Model file for the job. Use its own axes, mm. Coordinates: 2 decimals unless noted, no trailing zeros. Order: outer loops, then holes, each group sorted by start corner. A loop starts at its lowest first (then second) coordinate and runs counter-clockwise, first axis right, second up.
from build123d import *

# Parameters (mm, degrees)
F0_W     = 94.519034
F0_H     = 86.812686
F0_R     = 5.413518
F0_R_2   = 4.626995
F0_R_3   = 6.390639
F0_R_4   = 9.062056
F0_R_5   = 19.480322
F0_R_6   = 4.110136
F0_R_7   = 4.393433
F0_R_8   = 8.620442
F0_R_9   = 7.192681
F0_R_10  = 4.466697
F1_ANGLE = 45


with BuildPart() as f1:
    # F0 (on Front) → F1 (revolve)
    with BuildSketch(Plane.XZ):
        with Locations((-17.815083, 3.718389)):
            Rectangle(F0_W, F0_H)
        with Locations((-53.812075, -27.955186)):
            Circle(F0_R, mode=Mode.SUBTRACT)
        with Locations((-30.148292, -29.630704)):
            Circle(F0_R_2, mode=Mode.SUBTRACT)
        with Locations((11.945384, -26.993094)):
            Circle(F0_R_3, mode=Mode.SUBTRACT)
        with Locations((-4.236709, -16.035384)):
            Circle(F0_R_4, mode=Mode.SUBTRACT)
        with Locations((-29.292393, 7.944192)):
            Circle(F0_R_5, mode=Mode.SUBTRACT)
        with Locations((-57.312123, 32.896079)):
            Circle(F0_R_6, mode=Mode.SUBTRACT)
        with Locations((-41.277222, 36.766876)):
            Circle(F0_R_7, mode=Mode.SUBTRACT)
        with Locations((5.348549, 12.50712)):
            Circle(F0_R_8, mode=Mode.SUBTRACT)
        with Locations((-7.967654, 32.40367)):
            Circle(F0_R_9, mode=Mode.SUBTRACT)
        with Locations((10.63888, 32.776453)):
            Circle(F0_R_10, mode=Mode.SUBTRACT)
    revolve(axis=Axis((29.444434, 0, 3.718389), (0, 0, -1)), revolution_arc=F1_ANGLE)


solid = f1.part
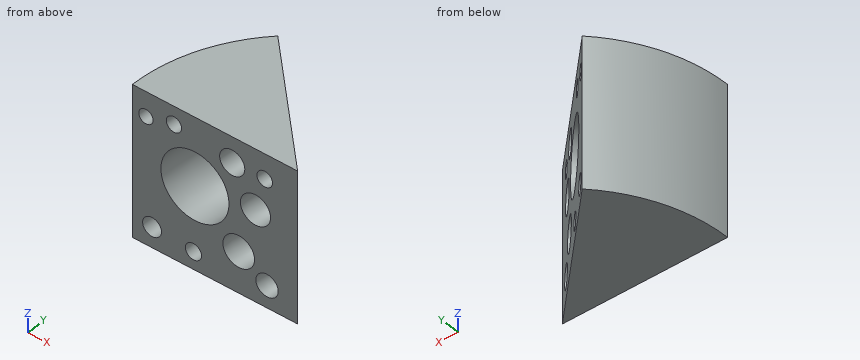
Q1. Probe line 1 (Z direction, x = 10, y = 4.5); line 2 (Z direction, x = 5, y = 9.5); line 3 (Z direction, x = -13, y = 9). List the from-to ranges inside material, lowest first.
Established:
line 1: z = -39.69 to -32.89, -21.09 to 4.94, 20.07 to 28.46, 37.09 to 47.12
line 2: z = -39.69 to -21.19, -10.88 to 4.15, 20.86 to 47.12
line 3: z = -39.69 to -4.05, 19.94 to 28.4, 36.41 to 47.12
Q2. Drop flat-ended pins along their axis: P1, Ø4, axis at y = 50.5, z = 6.5, coming from the +X side; P2, Ø5, axis at y = 19.5, z = 33, coming from the -X side; P3, Ø1.5, axis at x = -41, z = 17, coming from the +Y side. Give the stop position or say it passes through.
Established:
P1: stops at x = -28.45
P2: stops at x = -63.53
P3: stops at y = 63.85
Q3. Cut at D-D, the plane x = -23.5. Count the separate pieces of the cut face and the enclosed holes in it, plus the area to 3 significant figures.
Established:
separate pieces: 2
enclosed holes: 1
area: 2,440 mm2
Q4. Cut at A-A, the plane z = 14.5. List the corners of the cut face in (x, y), plus the area to 3 significant figures.
Established:
outline: (-65.07, 0) - (-47.64, 0) arc R77.08 cw to (-25.06, 54.5) - (-37.39, 66.84) arc R94.52 ccw to start; (-10.95, 0) - (-3.04, 0) arc R32.48 cw to (6.48, 22.97) - (0.88, 28.56) arc R40.39 ccw to start; (13.74, 0) - (29.44, 0) - (18.34, 11.11) arc R15.71 ccw to start
area: 1,500 mm2
Q5. Cut at C-C, the plane z = 0.5. List the corners of the cut face in (x, y).
Established:
outline: (-65.07, 0) - (-47.29, 0) arc R76.74 cw to (-24.82, 54.26) - (-37.39, 66.84) arc R94.52 ccw to start; (-11.29, 0) - (29.44, 0) - (0.64, 28.8) arc R40.73 ccw to start
Q6. Cut at B-B, the plane z = 35. List the corners of the cut face in (x, y).
Established:
outline: (-65.07, 0) - (-60.84, 0) arc R90.29 cw to (-34.4, 63.84) - (-37.39, 66.84) arc R94.52 ccw to start; (-53.78, 0) - (-45.3, 0) arc R74.74 cw to (-23.41, 52.85) - (-29.41, 58.85) arc R83.23 ccw to start; (-37.25, 0) - (-14.68, 0) arc R44.12 cw to (-1.75, 31.2) - (-17.72, 47.16) arc R66.7 ccw to start; (-1.26, 0) - (6.76, 0) arc R22.68 cw to (13.41, 16.04) - (7.73, 21.71) arc R30.7 ccw to start; (14.51, 0) - (29.44, 0) - (18.89, 10.56) arc R14.93 ccw to start
